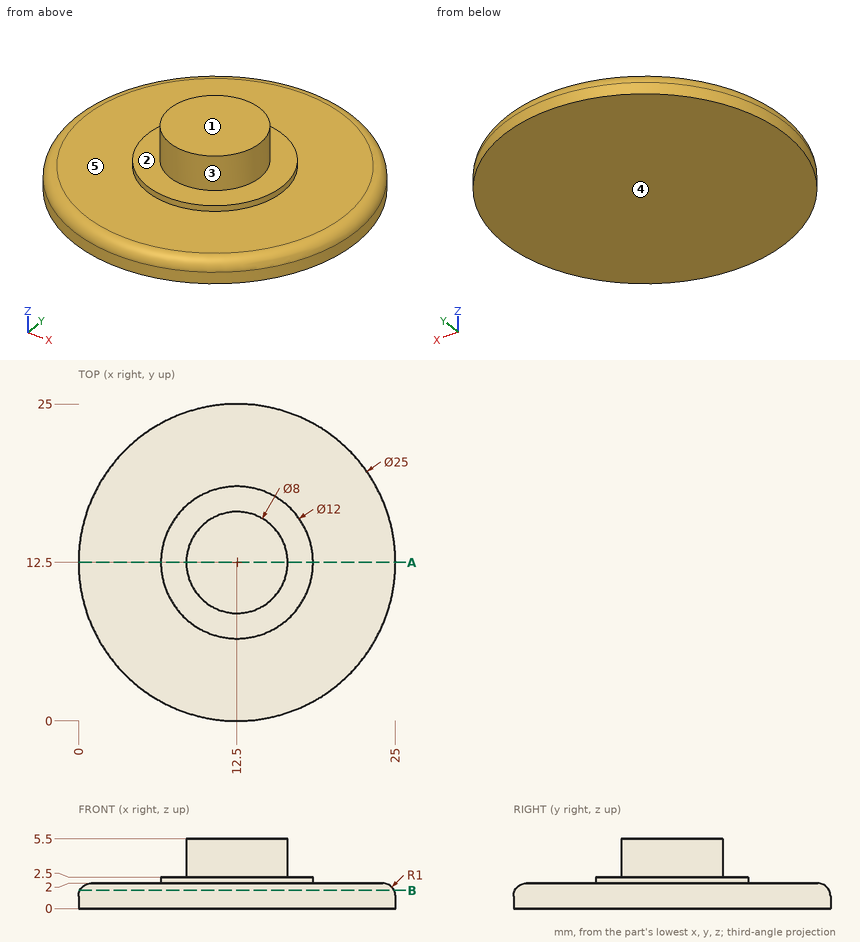
Part print with two shaded views. Sizes in mm from the minimum x, y, z corner. A direction names the side the tool comes from. Coordinates: 2 decimals unless noted, no trailing zeros. Loops run counter-clockwise (first coordinate to the right, second up) from the corner with the lowest first, then second, coordinate; pieces in that order, holes last. Notation, with made-up numbers: M 81.25,73 L 90.25,73 A17 ccw 90.25,91 Z; hole C 65.25,15 d8. An arc over 180 degrees is marked long. Use CSV: the item, a comma, the result in double quotes. Start each with the question number.
1. Band-saw the part on B-B, the plane z = 1.45. List the corners of the cut face in (x, y), then the cut area to 3 significant figures.
2. Probe probe 1 along Z at (x, y) = (7.25, 7); probe 2 along Z at (x, y) = (16, 14.5); probe 3 along Y at (x, z) = (12.75, 1). List the from-to ranges inside material, lowest first. Write a range as [from, to].
3. Band-saw the part on A-A, the plane y = 12.5. List the corners of the cut face in (x, z), then the cut area to 3 significant figures.
4. Tool access for the marked faces 1 and 2: list every direction of +Z, -Z, +X, -X, +Y, -Y with a clear straight run to the whole face (end or side of a thin tool).
5. Flat gauge pins, fed straight in: pin 1 (3 mm diameter, centred on y = 15.5, z = 3, fed in from -X); pin 2 (1 mm diameter, centred on x = 12, z = 2, fed in from +Y); pin 3 (1.5 mm diameter, centred on y = 11.5, z = 2, fed in from +X). Where does each tip first touch, or does it go through?
6. Two-plate mould, pull along Z, no slides. Class the marked faces 3, 4 and 5: pulls with the +Z half, pulls with the -Z half, needs draft (parallel to the pull), parting line crosses it, or undercut.
Entries:
1,outline,"C 12.5,12.5 d24.79"
1,area,"483 mm2"
2,probe 1,"z = [0, 2]"
2,probe 2,"z = [0, 2.5]"
2,probe 3,"y = [0, 25]"
3,outline,"M 0,0 L 25,0 L 25,1 A1 ccw 24,2 L 18.5,2 L 18.5,2.5 L 16.5,2.5 L 16.5,5.5 L 8.5,5.5 L 8.5,2.5 L 6.5,2.5 L 6.5,2 L 1,2 A1 ccw 0,1 Z"
3,area,"79.6 mm2"
4,face 1,"+Z, +X, -X, +Y, -Y"
4,face 2,"+Z"
5,pin 1,"stops at x = 0.44"
5,pin 2,"stops at y = 24.86"
5,pin 3,"stops at x = 24.94"
6,face 3,"needs draft"
6,face 4,"pulls with the -Z half"
6,face 5,"pulls with the +Z half"
